Geometry: final body of the model. Coordinates: model frame, mm. Face numbers are marked on the shaded views. A direction names the side the tool comes from. Give positions to 0.01 mm unless a question says otherwise; leave off trailing zeros. Write each loop counter-clockwise with the first axis right and the second up, starting at its lowest first coordinate (ties: lowest second). Pieces come first, ordered by that corner, then holes. Notation, with made-up numbers: (-39, 84.25) -> (8, 84.25) arc R24 ccw to (8, 103.25) -> close; hole circle Ø9 at (-23, 66). An arc over 180 degrees is marked (long way). Answer in a Markdown table with one row per item. Add a question column.
Item 1: Section query D-D on z = -92. Output: boundary loops of the cut face in (x, y).
Item 2: Section query C-C on y = 311. Output: boundary loops of the cut face in (x, z).
Item 3: Section query B-B on z = 254. Output: boundary loops of the cut face in (x, y), plus the area to 3 significant figures.
Item 4: Material intervals for probe 1 along X at (y, z) = (174, -762); probe 2 along Y at (x, z) = (-137.5, 252.5); probe 3 along Z at (x, y) = (-42, 355), sorted ascending. Write a range as from..to.
Item 5: Section query A-A on y = 149. Output: boundary loops of the cut face in (x, z).
Item 6: Access query for the marked faces 5, 6 and 7. Directions: +Z, -Z, +X, -X, +Y, -Y. A direction counts if a zero-diameter tool reaches every point of the face in a straight line with its end or side. Return the directions, or none.
Item 7: Draft query along Y for the marked faces 1, 2, 3 and 4. Return one class per face: +Y half, -Y half, draft (parallel to the pull), parting line (faces both ways), or undercut.
Item 8: First-contact query: P1, Ø2, axis at x = 317, z = -971, coming from the -Y side; P2, Ø12, axis at x = 356.5, y = 254, coming from the +Z side; P3, Ø6, axis at x = 40.5, y = -234.5, coming from the +Z side. Flat tips, straight axial feed; report the tip coordinate or a pass-through.
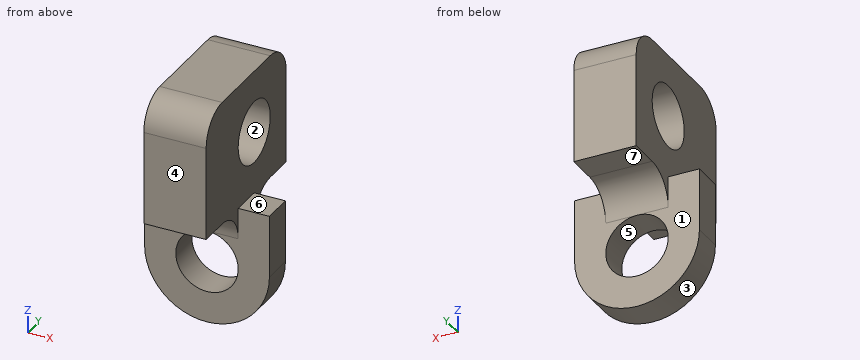
```python
from build123d import *

# Parameters (mm, degrees)
SKETCH1_R           = 254
BOSS_EXTRUDE2_DEPTH = 254
SKETCH3_R           = 254
BOSS_EXTRUDE3_DEPTH = 254


with BuildPart() as part:
    # Sketch1 → Boss-Extrude2 (new, symmetric)
    with BuildSketch(Plane(origin=(0, 0, 0), x_dir=(0, 0, -1), z_dir=(1, 0, 0))):
        with BuildLine():
            Line((-762, 609.6), (-762, -152.4))
            ThreePointArc((-762, -152.4), (-687.605122421, -332.005122421), (-508, -406.4))
            Line((-508, -406.4), (254, -406.4))
            Line((254, -406.4), (254, -152.4))
            ThreePointArc((254, -152.4), (328.394877579, 27.205122421), (508, 101.6))
            Line((508, 101.6), (254, 101.6))
            Line((254, 101.6), (254, 355.6))
            Line((254, 355.6), (508, 355.6))
            ThreePointArc((508, 355.6), (328.394877579, 429.994877579), (254, 609.6))
            Line((254, 609.6), (254, 863.6))
            Line((254, 863.6), (-508, 863.6))
            ThreePointArc((-508, 863.6), (-687.605122421, 789.205122421), (-762, 609.6))
        make_face()
        with Locations((-254, 355.6)):
            Circle(SKETCH1_R, mode=Mode.SUBTRACT)
    extrude(amount=BOSS_EXTRUDE2_DEPTH, both=True)

    # Sketch3 → Boss-Extrude3 (add)
    with BuildSketch(Plane(origin=(0, 101.6, 0), x_dir=(1, 0, 0), z_dir=(0, 1, 0))):
        with BuildLine():
            Line((-508, 254), (508, 254))
            Line((508, 254), (508, 762))
            ThreePointArc((508, 762), (0, 1270), (-508, 762))
            Line((-508, 762), (-508, 254))
        make_face()
        with Locations(Location((0, 762, 0), (0, 0, 270))):
            Circle(SKETCH3_R, mode=Mode.SUBTRACT)
    extrude(amount=BOSS_EXTRUDE3_DEPTH)


solid = part.part
```
Findings below:
| question | item | result |
|---|---|---|
| 1 | outline | (-254, -406.4) -> (254, -406.4) -> (254, 863.6) -> (-254, 863.6) -> close |
| 2 | outline | (-508, -762) arc R508 ccw to (508, -762) -> (508, -254) -> (254, -254) -> (254, 3.95) -> (-254, 3.95) -> (-254, -254) -> (-508, -254) -> close; (-254, 504.05) -> (254, 504.05) -> (254, 762) -> (-254, 762) -> close; hole circle Ø508 at (0, -762) |
| 3 | outline | (-254, -406.4) -> (254, -406.4) -> (254, 101.6) -> (-254, 101.6) -> close; (-254, 609.6) -> (254, 609.6) -> (254, 863.6) -> (-254, 863.6) -> close |
| 3 | area | 387,000 mm^2 |
| 4 | probe 1 | x = -508..-254, 254..508 |
| 4 | probe 2 | y = -406.4..101.6, 609.6..863.6 |
| 4 | probe 3 | z = -1268.26..-1012.5, -511.5..0, 508..762 |
| 5 | outline | (-508, -762) arc R508 ccw to (508, -762) -> (508, -254) -> (254, -254) -> (254, 106.24) -> (-254, 106.24) -> (-254, -254) -> (-508, -254) -> close; (-254, 401.76) -> (254, 401.76) -> (254, 762) -> (-254, 762) -> close; hole circle Ø508 at (0, -762) |
| 6 | face 5 | +Y, -Y |
| 6 | face 6 | +Z, +X, +Y, -Y |
| 6 | face 7 | -Z, +X, -X, +Y |
| 7 | face 1 | +Y half |
| 7 | face 2 | undercut |
| 7 | face 3 | draft |
| 7 | face 4 | -Y half |
| 8 | P1 | stops at y = 101.6 |
| 8 | P2 | stops at z = -254 |
| 8 | P3 | stops at z = 749.37 |
